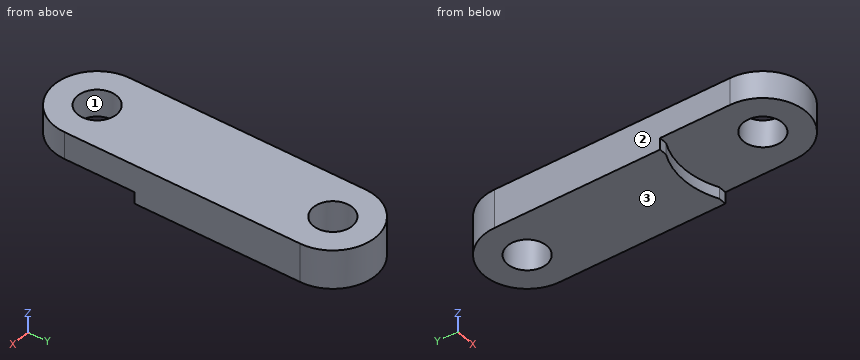
```python
from build123d import *

# Parameters (mm, degrees)
SKETCH1_R           = 5
BOSS_EXTRUDE1_DEPTH = 10
CUT_EXTRUDE1_DEPTH  = 3


with BuildPart() as part:
    # Sketch1 → Boss-Extrude1 (new body)
    with BuildSketch(Plane(origin=(0, 0, 0), x_dir=(0, 1, 0), z_dir=(0, 0, 1))):
        with BuildLine():
            Line((0, 11), (60, 11))
            ThreePointArc((60, 11), (71, 0), (60, -11))
            Line((60, -11), (0, -11))
            ThreePointArc((0, -11), (-11, 0), (0, 11))
        make_face()
        with Locations(Location((0, 0, 0), (0, 0, 270))):
            Circle(SKETCH1_R, mode=Mode.SUBTRACT)
        with Locations(Location((60, 0, 0), (0, 0, 270))):
            Circle(SKETCH1_R, mode=Mode.SUBTRACT)
    extrude(amount=BOSS_EXTRUDE1_DEPTH)

    # Sketch2 → Cut-Extrude1 (cut)
    with BuildSketch(Plane(origin=(0, 0, 0), x_dir=(1, 0, 0), z_dir=(0, 0, -1))):
        with BuildLine():
            Line((9, -17.860571099), (11, -17.860571099))
            Line((11, -17.860571099), (11, 0))
            ThreePointArc((11, 0), (0, 11), (-11, 0))
            Line((-11, 0), (-11, -17.860571099))
            Line((-11, -17.860571099), (-9, -17.860571099))
            ThreePointArc((-9, -17.860571099), (0, -20), (9, -17.860571099))
        make_face()
    extrude(amount=-CUT_EXTRUDE1_DEPTH, mode=Mode.SUBTRACT)


solid = part.part
```
Geometry: final body of the model. Coordinates: model frame, mm. Face numbers are marked on the shaded views. Coordinates: 2 decimals unless noted, no trailing zeros. Order: outer loops, then holes, each group sorted by start corner. A loop starts at its lowest first (then second) coordinate and runs counter-clockwise, first axis right, second up. Notation, with made-up numbers: M 77.25,54 L 89.25,54 A19 ccw 89.25,58 Z; hole C 65.5,74 d7. An arc over 180 degrees is marked long. Answer in a Markdown table with one row per item. Add a question column.
Q1. Section query A-A on x = 0. Return the cut outline in (y, z), and give its area (3 significant figures).
Q2. Section query D-D on z = 7.75. Return the cut outline in (x, y), and give its area (3 significant figures).
Q3. Line query: L1, parallel to Y at x = 0, z = 8; L2, parallel to Y at x = -4, z = 6.5; L3, parallel to Z at x = -9, y = 10. Output: solid intervals per line, ascending.
Q4. Section query C-C on y = 1. Return the cut outline in (x, z), and give its area (3 significant figures).
Q5. Mould query, pull axis X, two halves, no side actions, for the marked faces 1, 2 and 3. Classes: released by +X, released by -X, zero draft, split by the parting line, or undercut.
Q6. Section query B-B on z = 1.75. Return the cut outline in (x, y).
Q7. Contact query for flat-ended pins moving along their axis: P1, Ø2, axis at x = -10, z = 1, coming from the -Y side; P2, Ø6, axis at x = -5, z = 7.5, coming from the +Y side; P3, Ø1.5, axis at x = 1, z = 6, coming from the +Y side; P4, Ø9, axis at x = 0, y = 0, coming from the -Z side. Output: stop coordinate, or through.
Completed:
| question | item | result |
|---|---|---|
| 1 | outline | M -11,3 L -5,3 L -5,10 L -11,10 Z; M 5,3 L 20,3 L 20,0 L 55,0 L 55,10 L 5,10 Z; M 65,0 L 71,0 L 71,10 L 65,10 Z |
| 1 | area | 557 mm2 |
| 2 | outline | M -11,0 A11 ccw 11,0 L 11,60 A11 ccw -11,60 Z; hole C 0,0 d10; hole C 0,60 d10 |
| 2 | area | 1,540 mm2 |
| 3 | L1 | y = -11 to -5, 5 to 55, 65 to 71 |
| 3 | L2 | y = -10.25 to -3, 3 to 57, 63 to 70.25 |
| 3 | L3 | z = 3 to 10 |
| 4 | outline | M -11,3 L -4.9,3 L -4.9,10 L -11,10 Z; M 4.9,3 L 11,3 L 11,10 L 4.9,10 Z |
| 4 | area | 85.4 mm2 |
| 5 | face 1 | undercut |
| 5 | face 2 | released by -X |
| 5 | face 3 | zero draft |
| 6 | outline | M -11,17.86 L -9,17.86 A20 cw 9,17.86 L 11,17.86 L 11,60 A11 ccw -11,60 Z; hole C 0,60 d10 |
| 7 | P1 | stops at y = 17.86 |
| 7 | P2 | stops at y = 70.82 |
| 7 | P3 | stops at y = 71 |
| 7 | P4 | passes through |
